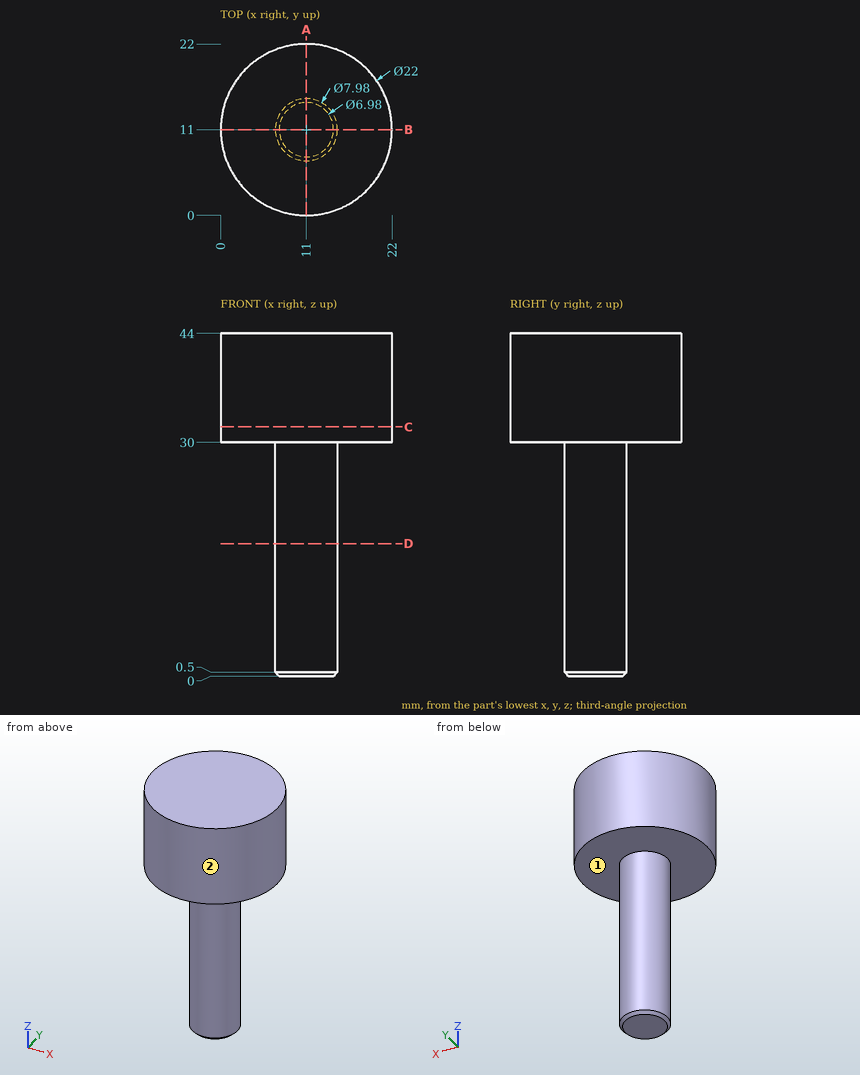
Answer from the drawing. Dimensions are ordinates in mm from the lowest x, y and z of the part. A direction names the side the tool comes from. Give positions to 0.01 mm unless a question says otherwise; leave off trailing zeros. Order: outer loops, then holes, each group sorted by start corner. A loop starts at its lowest first (then second) coordinate and runs counter-clockwise, first axis right, second up. Notation, with made-up numbers: (-19.75, -25) -> (19.25, -25) arc R21 ccw to (19.25, -19) -> close; hole circle Ø10 at (40, 35). An arc over 180 degrees is marked (long way). Answer as a JSON object with one key per item and string values. Group by question number.
1. Section A-A on x = 11 is taken. Determine the outline of the cut face in (y, z), plus the area to 3 significant figures.
2. Section C-C on z = 32 is taken. Determine the outline of the cut face in (x, y), plus the area to 3 significant figures.
3. Section D-D on z = 17 is taken. Determine the outline of the cut face in (x, y).
4. Flat-ended cylindrical pins translate along their axes: pin 1 Ø1 at (y, z) = (7, 28.5) entering from -X; pin 2 Ø1 at (x, z) = (18.5, 33) entering from +Y; pin 3 Ø8 at (y, z) = (9, 23) entering from +X. Find the tip coordinate at first contact, or state that the pin passes through.
5. A tool of negligible diameter and unlimited length cuts with its end or side. For the marked faces 1 and 2, from which of +Z, -Z, +X, -X, +Y, -Y can it reach the whole face along a straight path? Write none if from no direction.
6. Consider line 1 along Z through (x, y) = (5.75, 15); line 2 along Y through (x, z) = (11, 37.5); line 3 along Y through (x, z) = (14.5, 20.5). Determine where each line is inside the solid, lowest interval first. Write a range as [from, to].
Result sheet:
{
 "1": {"outline": "(0, 30) -> (7.01, 30) -> (7.01, 0.5) -> (7.51, 0) -> (14.49, 0) -> (14.99, 0.5) -> (14.99, 30) -> (22, 30) -> (22, 44) -> (0, 44) -> close", "area": "547 mm^2"},
 "2": {"outline": "circle Ø22 at (11, 11)", "area": "380 mm^2"},
 "3": {"outline": "circle Ø7.98 at (11, 11)"},
 "4": {"pin 1": "stops at x = 9.08", "pin 2": "stops at y = 19.49", "pin 3": "stops at x = 14.99"},
 "5": {"face 1": "-Z", "face 2": "+Z, -Z"},
 "6": {"line 1": "z = [30, 44]", "line 2": "y = [0, 22]", "line 3": "y = [9.08, 12.92]"}
}
